The drawing under review shows one solid part. Ordinate dimensions are in mm from its lowest x, y, z. A direction names the side the tool comes from. Round coordinates to 2 decimals unless told otherwise and drop trailing zeros. Order: outer loops, then holes, each group sorted by start corner. A loop starts at its lowest first (then second) coordinate and runs counter-clockwise, first axis right, second up.
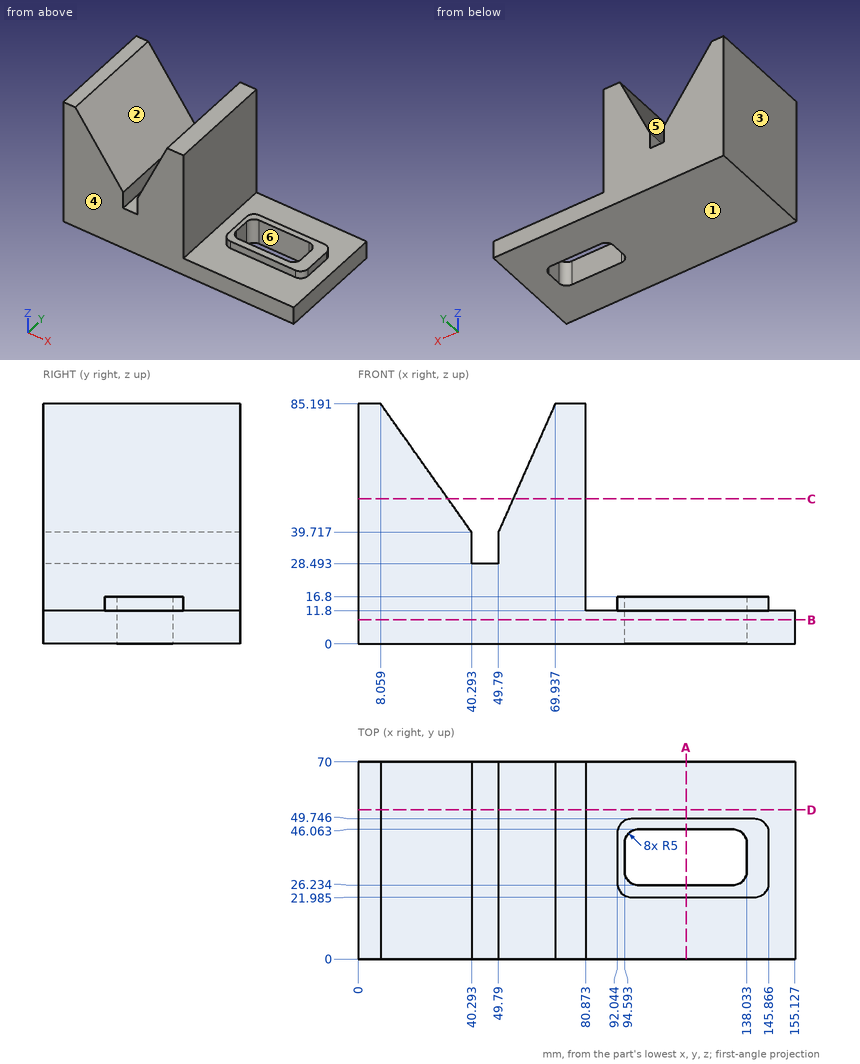
Q1. Tool access review of the marked faces 4, 5 and 6: name each direction out of +Z, -Z, +X, -X, +Y, -Y from which nothing blocks a thin tool from reaching the whole face with its end or side.
Q2. Take a section at C-C, the plane z = 51.5. State the section outline as (x, y) points, plus the area to 3 significant figures.
Q3. Take a section at D-D, the plane y = 53. State the section outline as (x, z) points.
Q4. Mouldability with a two-part tool opening along X and no side actions: class the marked faces 1, 2 and 3 as +X half, -X half, draft (parallel to the pull), parting line (faces both ways), or undercut.
Q5. Clearance check with flat-ended pins moving along their axes: pin 1 (2 mm diameter, centred on y = 22.5, z = 61, fed in from +X); pin 2 (21 mm diameter, centred on x = 110, y = 18.5, fed in from +Z); pin 3 (1.5 mm diameter, centred on x = 52.5, y = 46, fed in from +Z) (1 decimal). State where each tip first meets the part, or that it passes through.
Q6. Take a section at A-A, the plane x = 116.5. State the section outline as (y, z) points (1 decimal).
Q7. Wall thickness on line 1 (X direction, y = 30, z = 35.5); line 2 (X direction, y = 38.5, z = 11.5); line 3 (X direction, y = 5.5, z = 24.5): over which ranges is each line inside the solid? List them lowest first.
Q8. Take a section at B-B, the plane z = 8.5. State the section outline as (x, y) points (1 decimal), plus the area to 3 significant figures.
Working result:
1. face 4: +Z, -Z, +X, -X, -Y
1. face 5: +Z, +Y, -Y
1. face 6: +Z, -Z
2. outline: (0, 0) - (31.94, 0) - (31.94, 70) - (0, 70) - close; (55.01, 0) - (80.87, 0) - (80.87, 70) - (55.01, 70) - close
2. area: 4,050 mm2
3. outline: (0, 0) - (155.13, 0) - (155.13, 11.8) - (80.87, 11.8) - (80.87, 85.19) - (69.94, 85.19) - (49.79, 39.72) - (49.79, 28.49) - (40.29, 28.49) - (40.29, 39.72) - (8.06, 85.19) - (0, 85.19) - close
4. face 1: draft
4. face 2: undercut
4. face 3: -X half
5. pin 1: stops at x = 80.87
5. pin 2: stops at z = 16.8
5. pin 3: stops at z = 47.5
6. outline: (0, 0) - (26.2, 0) - (26.2, 16.8) - (22, 16.8) - (22, 11.8) - (0, 11.8) - close; (46.1, 0) - (70, 0) - (70, 11.8) - (49.7, 11.8) - (49.7, 16.8) - (46.1, 16.8) - close
7. line 1: x = 0 to 40.29, 49.79 to 80.87
7. line 2: x = 0 to 94.59, 138.03 to 155.13
7. line 3: x = 0 to 80.87
8. outline: (0, 0) - (155.1, 0) - (155.1, 70) - (0, 70) - close; hole (94.6, 31.2) arc R5 ccw to (99.6, 26.2) - (133, 26.2) arc R5 ccw to (138, 31.2) - (138, 41.1) arc R5 ccw to (133, 46.1) - (99.6, 46.1) arc R5 ccw to (94.6, 41.1) - close
8. area: 10,000 mm2
